from build123d import *

# Parameters (mm, degrees)
SKETCH1_W           = 75
SKETCH1_H           = 40
BOSS_EXTRUDE1_DEPTH = 2.5
CUT_EXTRUDE1_DEPTH  = 10
SKETCH2_3_W         = 8.2
SKETCH2_3_H         = 7.4
BOSS_EXTRUDE2_DEPTH = 23.814
FILLET1_R           = 3.25
FILLET2_R           = 3


with BuildPart() as part:
    # Sketch1 → Boss-Extrude1 (new body)
    with BuildSketch(Plane.XY):
        Rectangle(SKETCH1_W, SKETCH1_H)
    extrude(amount=BOSS_EXTRUDE1_DEPTH)

    # Sketch2 → Cut-Extrude1 (cut)
    with BuildSketch(Plane.XY):
        Polygon((12.9, -11.2), (12.9, 20), (-12.9, 20), (-12.9, -11.2), (-4.1, -11.2), (-4.1, -3.8), (4.1, -3.8), (4.1, -11.2), align=None)
    extrude(amount=CUT_EXTRUDE1_DEPTH, mode=Mode.SUBTRACT)

    # Sketch2<3> → Boss-Extrude2 (add)
    with BuildSketch(Plane.XY):
        with Locations((0, -7.5)):
            Rectangle(SKETCH2_3_W, SKETCH2_3_H)
    extrude(amount=-BOSS_EXTRUDE2_DEPTH)

    # Fillet1
    fillet1_edges = [part.edges().sort_by_distance(p)[0] for p in [
        (-12.9, 20, 1.25),
        (-12.9, -11.2, 1.25),
        (0, -3.8, 2.5),
        (0, -11.2, 0),
        (12.9, -11.2, 1.25),
        (12.9, 20, 1.25),
        (0, -11.2, -23.814),
    ]]
    fillet(fillet1_edges, radius=FILLET1_R)

    # Fillet2
    fillet2_edges = [part.edges().sort_by_distance(p)[0] for p in [
        (-4.1, -11.2, 1.25),
        (4.1, -11.2, 1.25),
    ]]
    fillet(fillet2_edges, radius=FILLET2_R)


solid = part.part
Source: CAD feature listing. Evaluate the final solid. Frame: model axes, mm. A direction names the side the tool comes from. Round coordinates to 2 decimals unless told otherwise and drop trailing zeros. Order: outer loops, then holes, each group sorted by start corner. A loop starts at its lowest first (then second) coordinate and runs counter-clockwise, first axis right, second up. Notation, with made-up numbers: (56.5, -3) - (107.5, -3) arc R18 cw to (107.5, 1) - close; hole circle Ø3 at (-19.75, -35). An arc over 180 degrees is marked (long way). Use a Markdown table: item, result. Add a question column.
1. Section query A-A (y = -1.5). Return the cut outline in (x, z).
2. Section query D-D (x = 26). Return the cut outline in (y, z).
3. Section query B-B (z = -2). Return the cut outline in (x, y), then the cut area to 3 significant figures.
4. Set-up query: faces 1 (the cylindrical face through (-13.827, 19.023, 1.268)), 2 (the flat face through (0, -3.8, -12)), 3 (the flat face through (0, -11.2, -12)). Return all of +Z, -Z, +X, -X, +Y, -Y with unobstructed straight access to the full face (end or side cutting, diameter ignored); none if empty.
5. Section query C-C (y = -12.5). Return the cut outline in (x, z), then the cut area to 3 significant figures.
6. First-contact query: pin 1 (1.5 mm diameter, centred on y = 9.5, z = -2, fed in from -X); pin 2 (5.5 mm diameter, centred on y = -8.5, z = -10, fed in from -X); pin 3 (6.5 mm diameter, centred on x = 1, z = -11, fed in from +Y); pin 4 (3 mm diameter, centred on x = -8, z = 1.5, fed in from +Y). Flat tips, straight axial feed; report the tip coordinate or a pass-through.
7. Line query: probe 1 along Z at (x, y) = (12, -17); probe 2 along X at (y, z) = (-4, -2). Output: solid intervals per line, ascending.
8. Mould query, pull axis X, two halves, no side actions, for faces 4 (the flat face through (-1, -20, 1)), 5 (the flat face through (-37.5, 0, 1)), 6 (the flat face through (-12.9, 5, 1)). Classes: +X half, -X half, draft (parallel to the pull), parting line (faces both ways), or undercut.
Derived:
| question | item | result |
|---|---|---|
| 1 | outline | (-37.5, 0) - (-12.9, 0) - (-12.9, 2.5) - (-37.5, 2.5) - close; (12.9, 0) - (37.5, 0) - (37.5, 2.5) - (12.9, 2.5) - close |
| 2 | outline | (-20, 0) - (20, 0) - (20, 2.5) - (-20, 2.5) - close |
| 3 | outline | (-4.1, -11.45) - (4.1, -11.45) - (4.1, -3.8) - (-4.1, -3.8) - close |
| 3 | area | 62.7 mm2 |
| 4 | face 1 | +Z, -Z, +Y |
| 4 | face 2 | +Z, -Z, +X, -X, +Y |
| 4 | face 3 | -Z, +X, -X, -Y |
| 5 | outline | (-37.5, 0) - (-4.1, 0) - (-4.1, -0.65) - (4.1, -0.65) - (4.1, 0) - (37.5, 0) - (37.5, 2.5) - (-37.5, 2.5) - close |
| 5 | area | 193 mm2 |
| 6 | pin 1 | through |
| 6 | pin 2 | x = -4.1 |
| 6 | pin 3 | y = -3.8 |
| 6 | pin 4 | y = -11.14 |
| 7 | probe 1 | 0 to 2.5 |
| 7 | probe 2 | -4.1 to 4.1 |
| 8 | face 4 | draft |
| 8 | face 5 | -X half |
| 8 | face 6 | undercut |
